```python
from build123d import *

# Parameters (mm, degrees)
SKETCH2_W                                  = 105
SKETCH2_H                                  = 85
BOSS_EXTRUDE1_DEPTH                        = 10
CASTER_MOUNTING_HOLES_TZPPED_HOLES_M8X1_D  = 6.8
CENTER_PROFILE_CS_HOLE_M8X1_25_D           = 8
CENTER_PROFILE_CS_HOLE_M8X1_25_DEPTH       = 10
CENTER_PROFILE_CS_HOLE_M8X1_25_CSINK_D     = 18
CENTER_PROFILE_CS_HOLE_M8X1_25_CSINK_ANGLE = 90
CENTER_PROFILE_CS_HOLE_M8X1_25_TIP         = 2.403442476
FILLET1_R                                  = 7


with BuildPart() as part:
    # Sketch2 → Boss-Extrude1 (new body)
    with BuildSketch(Plane(origin=(0, 0, 0), x_dir=(1, 0, 0), z_dir=(0, 1, 0))):
        Rectangle(SKETCH2_W, SKETCH2_H)
    extrude(amount=BOSS_EXTRUDE1_DEPTH)

    # caster mounting holes tzpped holes, m8x1.25 (through all)
    with Locations(Plane(origin=(0, 10, 0), x_dir=(1, 0, 0), z_dir=(0, 1, 0))):
        with Locations((-41.25, 31.25), (-41.25, -31.25), (41.25, -31.25), (41.25, 31.25)):
            Hole(CASTER_MOUNTING_HOLES_TZPPED_HOLES_M8X1_D / 2)

    # center profile cs hole, m8x1.25
    with Locations(Plane(origin=(0, 0, 0), x_dir=(-1, 0, 0), z_dir=(0, -1, 0))):
        with Locations((0, 0)):
            CounterSinkHole(CENTER_PROFILE_CS_HOLE_M8X1_25_D / 2, CENTER_PROFILE_CS_HOLE_M8X1_25_CSINK_D / 2, depth=CENTER_PROFILE_CS_HOLE_M8X1_25_DEPTH, counter_sink_angle=CENTER_PROFILE_CS_HOLE_M8X1_25_CSINK_ANGLE)
            with Locations((0, 0, -(CENTER_PROFILE_CS_HOLE_M8X1_25_DEPTH + CENTER_PROFILE_CS_HOLE_M8X1_25_TIP / 2))):  # 118° drill point
                Cone(0, CENTER_PROFILE_CS_HOLE_M8X1_25_D / 2, CENTER_PROFILE_CS_HOLE_M8X1_25_TIP, mode=Mode.SUBTRACT)

    # Fillet1
    fillet1_edges = [part.edges().sort_by_distance(p)[0] for p in [
        (52.5, 5, 42.5),
        (-52.5, 5, 42.5),
        (-52.5, 5, -42.5),
        (52.5, 5, -42.5),
    ]]
    fillet(fillet1_edges, radius=FILLET1_R)


solid = part.part
```
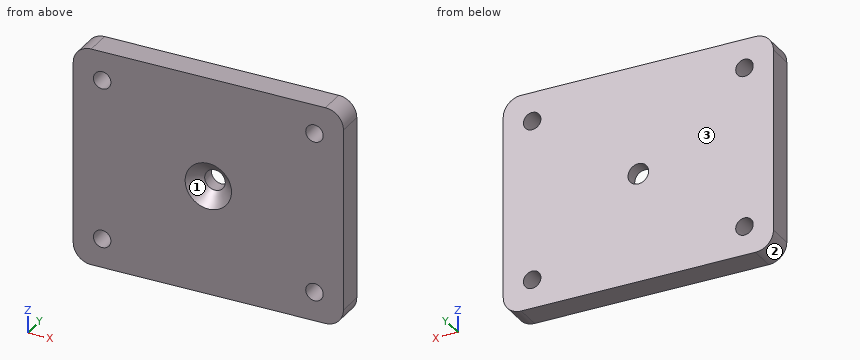
Verification items for the finished model (mm, model axes). Face numbers are marked on the shaded views. Round coordinates to 2 decimals unless told otherwise and drop trailing zeros. Loops run counter-clockwise (first coordinate to the right, second up) from the corner with the lowest first, then second, coordinate; pieces in that order, holes last. Notation, with made-up numbers: (-11.5, -6.75) -> (32.5, -6.75) arc R24 cw to (32.5, 30.25) -> close; hole circle Ø2 at (14.5, -21.5). An arc over 180 degrees is marked (long way). Answer as a JSON object with one key per item and string values.
Q1. Section check A-A (y = 1.5). Record the boundary of the cut face in (x, z).
Data:
{"outline": "(-52.5, -35.5) arc R7 ccw to (-45.5, -42.5) -> (45.5, -42.5) arc R7 ccw to (52.5, -35.5) -> (52.5, 35.5) arc R7 ccw to (45.5, 42.5) -> (-45.5, 42.5) arc R7 ccw to (-52.5, 35.5) -> close; hole circle Ø6.8 at (-41.25, -31.25); hole circle Ø6.8 at (-41.25, 31.25); hole circle Ø15 at (0, 0); hole circle Ø6.8 at (41.25, -31.25); hole circle Ø6.8 at (41.25, 31.25)"}
Q2. Scan lines: line 1 (X direction, y = 2.5, z = 31.25); line 2 (Z direction, x = 41.25, y = 7.5); line 3 (Z direction, x = 0, y = 6.4). Record each from-to range of solid material in increasing order. Write a range as from..to.
Data:
{"line 1": "x = -52.5..-44.65, -37.85..37.85, 44.65..52.5", "line 2": "z = -42.5..-34.65, -27.85..27.85, 34.65..42.5", "line 3": "z = -42.5..-4, 4..42.5"}
Q3. Draft check along Z on the marked faces 1, 2 and 3. Enter one of: pulls with the +Z half, pulls with the -Z half, needs draft (parallel to the pull), parting line crosses it, or undercut.
Data:
{"face 1": "undercut", "face 2": "pulls with the -Z half", "face 3": "needs draft"}
Q4. Section check D-D (x = 41.25). Record the boundary of the cut face in (y, z), then the cut area to 3 significant figures.
Data:
{"outline": "(0, -42.5) -> (10, -42.5) -> (10, -34.65) -> (0, -34.65) -> close; (0, -27.85) -> (10, -27.85) -> (10, 27.85) -> (0, 27.85) -> close; (0, 34.65) -> (10, 34.65) -> (10, 42.5) -> (0, 42.5) -> close", "area": "714 mm2"}
Q5. Go/stop test with a flat-tipped pin: P1, Ø6, axis at x = 41.25, z = -31.25, coming from the -Y side. Record where the tip stops, or that it passes through.
Data:
{"P1": "passes through"}
Q6. Section check C-C (z = 0). Record the boundary of the cut face in (x, y), then the cut area to 3 significant figures.
Data:
{"outline": "(-52.5, 0) -> (-9, 0) -> (-4, 5) -> (-4, 10) -> (-52.5, 10) -> close; (4, 5) -> (9, 0) -> (52.5, 0) -> (52.5, 10) -> (4, 10) -> close", "area": "945 mm2"}
Q7. Section check B-B (x = 0). Record the boundary of the cut face in (y, z).
Data:
{"outline": "(0, -42.5) -> (10, -42.5) -> (10, -4) -> (5, -4) -> (0, -9) -> close; (0, 9) -> (5, 4) -> (10, 4) -> (10, 42.5) -> (0, 42.5) -> close"}
